Input: dimensioned drawing with shaded views. Units: mm. Origin: part minimum x, y, z. A direction names the side the tool comes from. Coordinates: 2 decimals unless noted, no trailing zeros. Loops run counter-clockwise (first coordinate to the right, second up) from the corner with the lowest first, then second, coordinate; pieces in that order, holes last. Notation, with made-up numbers: (55.5, 6) - (80.5, 6) arc R15 cw to (80.5, 35) - close; hole circle Ø2 at (-34, 51.25). An arc over 180 degrees is marked (long way). Put each result on its own line as item: value. Start each with the question number.
1) Material intervals for line 1 along Y through (x, z) = (13, 0.5); line 2 along Y through (x, z) = (17.25, 2.5) (1 decimal); line 3 along Y through (x, z) = (7.5, 3.85) (1 decimal), sorted ascending. Write a range as from..to.
2) Reachability of the marked faces 1, 2 and 3 from +Z, -Z, +X, -X, +Y, -Y: full face, straight path, thin tool, end or side. Return the list, or none.
3) Draft query along Y for the marked faces 4, 5, 6 and 7. Return one class per face: +Y half, -Y half, draft (parallel to the pull), parting line (faces both ways), or undercut.
4) Section A-A on x = 11.75. Output: boundary loops of the cut face in (y, z) (1 decimal).
5) Section D-D on x = 7.5. Output: boundary loops of the cut face in (y, z).
6) Section C-C on y = 22. Output: boundary loops of the cut face in (x, z), and give its area (3 significant figures).
7) Section B-B on z = 3. Output: boundary loops of the cut face in (x, y).
8) Contact query for flat-ended pins moving along their axis: pin 1 Ø6.5 at (x, y) = (11.5, 22) entering from +Z; pin 2 Ø9 at (x, y) = (7.33, 19.14) entering from +Z. Output: stop coordinate, or through.
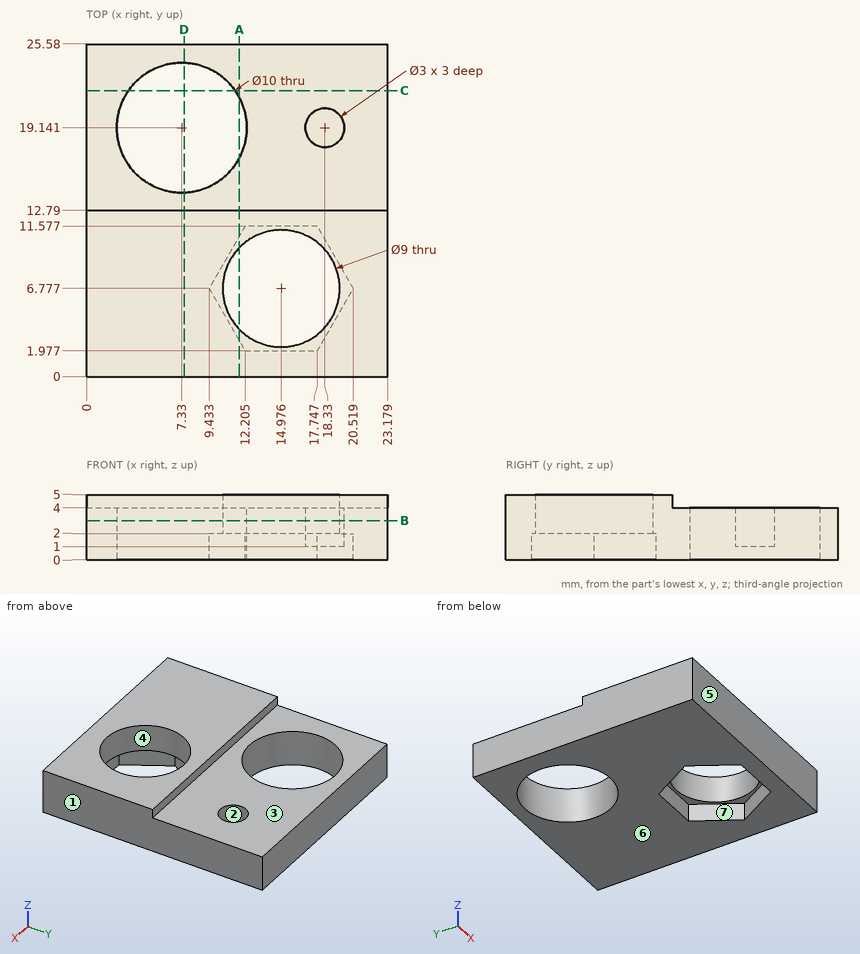
Answer block:
1. line 1: y = 0..1.98, 11.58..25.58
1. line 2: y = 0..2.9, 10.7..18.1, 20.2..25.6
1. line 3: y = 0..14.1, 24.1..25.6
2. face 1: +Z, -Z, +X, +Y, -Y
2. face 2: +Z
2. face 3: +Z, +X, -X, +Y
3. face 4: undercut
3. face 5: -Y half
3. face 6: draft
3. face 7: undercut
4. outline: (0, 0) - (2.8, 0) - (2.8, 2) - (3.6, 2) - (3.6, 5) - (0, 5) - close; (9.9, 2) - (10.8, 2) - (10.8, 0) - (16.8, 0) - (16.8, 4) - (12.8, 4) - (12.8, 5) - (9.9, 5) - close; (21.5, 0) - (25.6, 0) - (25.6, 4) - (21.5, 4) - close
5. outline: (0, 0) - (14.14, 0) - (14.14, 4) - (12.79, 4) - (12.79, 5) - (0, 5) - close; (24.14, 0) - (25.58, 0) - (25.58, 4) - (24.14, 4) - close
6. outline: (0, 0) - (3.23, 0) - (3.23, 4) - (0, 4) - close; (11.43, 0) - (23.18, 0) - (23.18, 4) - (11.43, 4) - close
6. area: 59.9 mm²
7. outline: (0, 0) - (23.18, 0) - (23.18, 25.58) - (0, 25.58) - close; hole circle Ø10 at (7.33, 19.14); hole circle Ø9 at (14.98, 6.78); hole circle Ø3 at (18.33, 19.14)
8. pin 1: stops at z = 4
8. pin 2: passes through
